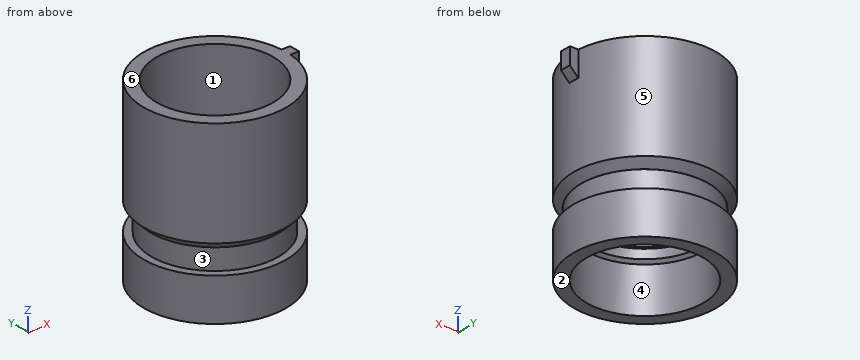
```python
from build123d import *

# Parameters (mm, degrees)
F0_R         = 17.1
F0_R_2       = 14
F1_DEPTH     = 10.2
F2_R         = 15.275
F2_R_2       = 14
F2_R_3       = 13.275
F3_DEPTH     = 5
F4_R         = 17.1
F4_R_2       = 15.275
F4_R_3       = 14
F5_DEPTH     = 27.1
F6_S5_R      = 14
F6_T6_DEPTH  = 22
F6_S11_R     = 14
F6_T12_DEPTH = 22
F7_SIZE      = 1.8
F9_DEPTH     = 6
F10_SIZE     = 1.99999


# Not quite as in the source:
# - a fillet or chamfer that OpenCascade refuses, or shapes differently, is made with other operations: its cross-section is extruded or revolved along the edge and cut away or added
# - a fillet or chamfer is up to 0.001 mm smaller than in the source, because OpenCascade refuses the exact size


with BuildPart() as f1:
    # F0 (on Top) → F1 (new body)
    with BuildSketch(Plane.XY):
        Circle(F0_R)
        Circle(F0_R_2, mode=Mode.SUBTRACT)
    extrude(amount=F1_DEPTH)

    # F2 (on face) → F3 (join)
    with BuildSketch(Plane.XY.offset(10.2)):
        Circle(F2_R)
        Circle(F2_R_2, mode=Mode.SUBTRACT)
        Circle(F2_R_2)
        Circle(F2_R_3, mode=Mode.SUBTRACT)
    extrude(amount=F3_DEPTH)

    # F4 (on face) → F5 (join)
    with BuildSketch(Plane.XY.offset(15.2)):
        Circle(F4_R)
        Circle(F4_R_2, mode=Mode.SUBTRACT)
        Circle(F4_R_2)
        Circle(F4_R_3, mode=Mode.SUBTRACT)
    extrude(amount=F5_DEPTH)

    # F6: chamfer of 1.4 on 2 edges, made by hand


with BuildPart() as f6_tool2:
    # F6_s3 → F6_t4 (revolve)
    with BuildSketch(Plane.XZ):
        Polygon((14.675, 10.2), (13.275, 11.6), (13.275, 10.2), align=None)
    revolve(axis=Axis((0, 0, 10.2), (0, 0, 1)))

    # F6_s5 → F6_t6 (intersect, symmetric)
    with BuildSketch(Plane.XY.offset(10.9)):
        Circle(F6_S5_R)
    extrude(amount=F6_T6_DEPTH, both=True, mode=Mode.INTERSECT)


with BuildPart() as f1_1:
    add(f1.part)

    # F6_t1: cut F6_tool2
    add(f6_tool2.part, mode=Mode.SUBTRACT)


with BuildPart() as f6_tool8:
    # F6_s9 → F6_t10 (revolve)
    with BuildSketch(Plane.XZ):
        Polygon((13.275, 13.8), (14.675, 15.2), (13.275, 15.2), align=None)
    revolve(axis=Axis((0, 0, 15.2), (0, 0, 1)))

    # F6_s11 → F6_t12 (intersect, symmetric)
    with BuildSketch(Plane.XY.offset(14.5)):
        Circle(F6_S11_R)
    extrude(amount=F6_T12_DEPTH, both=True, mode=Mode.INTERSECT)


with BuildPart() as f1_2:
    add(f1_1.part)

    # F6_t7: cut F6_tool8
    add(f6_tool8.part, mode=Mode.SUBTRACT)

    # F7
    f7_edges = [f1_2.edges().sort_by_distance(p)[0] for p in [
        (-17.1, 0, 15.2),
    ]]
    chamfer(f7_edges, length=F7_SIZE)

    # F8 (on face) → F9 (join)
    with BuildSketch(Plane.XY.offset(42.3)):
        with BuildLine():
            ThreePointArc((17.0505131888, 1.3), (17.0876238185, 0.6504707804), (17.1, 0))
            Line((17.1, 0), (19.1, 0))
            Line((19.1, 0), (19.1, 1.3))
            Line((19.1, 1.3), (17.0505131888, 1.3))
        make_face()
        with BuildLine():
            Line((19.1, 0), (17.1, 0))
            ThreePointArc((17.1, 0), (17.0876238185, -0.6504707804), (17.0505131888, -1.3))
            Line((17.0505131888, -1.3), (19.1, -1.3))
            Line((19.1, -1.3), (19.1, 0))
        make_face()
        with BuildLine():
            Line((17.1, 0), (17.0505131888, 0))
            Line((17.0505131888, 0), (17.0505131888, -1.3))
            ThreePointArc((17.0505131888, -1.3), (17.0876238185, -0.6504707804), (17.1, 0))
        make_face()
        with BuildLine():
            Line((17.0505131888, 1.3), (17.0505131888, 0))
            Line((17.0505131888, 0), (17.1, 0))
            ThreePointArc((17.1, 0), (17.0876238185, 0.6504707804), (17.0505131888, 1.3))
        make_face()
    extrude(amount=-F9_DEPTH)

    # F10 (size 2 in the source; OpenCascade refuses exactly that, so slightly less here)
    f10_edges = [f1_2.edges().sort_by_distance(p)[0] for p in [
        (19.1, 0, 36.3),
    ]]
    chamfer(f10_edges, length=F10_SIZE)


solid = f1_2.part
```
The model under review builds one solid part; all positions refer to its coordinate system, in mm. Face numbers are marked on the shaded views. A direction names the side the tool comes from. Round coordinates to 2 decimals unless told otherwise and drop trailing zeros. Loops run counter-clockwise (first coordinate to the right, second up) from the corner with the lowest first, then second, coordinate; pieces in that order, holes last. Notation, with made-up numbers: M 46,-14.75 L 60,-14.75 A26 ccw 60,22.25 Z; hole C -15.75,13 d1. An arc over 180 degrees is marked long. Put each result on its own line as item: value.
Q1. Machinability: for the marked faces 1, 2 and 3, which of the approach directions +Z, -Z, +X, -X, +Y, -Y give a long, thin tool a straight path to every point of the face, cutting with its end or side? Answer none if there is none.
Result set:
face 1: +Z
face 2: -Z, +X, -X, +Y, -Y
face 3: none
Q2. Consider section A-A, the plane x = 0. Give the boundary of the cut face in (y, z) (3 decimals), then the cut area to 3 significant figures.
Result set:
outline: M -17.1,0 L -14,0 L -14,10.875 L -13.275,11.6 L -13.275,13.8 L -14,14.525 L -14,42.3 L -17.1,42.3 L -17.1,17 L -15.3,15.2 L -15.275,15.2 L -15.275,10.2 L -17.1,10.2 Z; M 13.275,11.6 L 14,10.875 L 14,0 L 17.1,0 L 17.1,10.2 L 15.275,10.2 L 15.275,15.2 L 15.3,15.2 L 17.1,17 L 17.1,42.3 L 14,42.3 L 14,14.525 L 13.275,13.8 Z
area: 245 mm²
Q3. Mouldability with a two-part tool opening along Y and no side actions: class the marked faces 4, 5 and 6 as released by +Y, released by -Y, zero draft, split by the parting line, or undercut.
Result set:
face 4: undercut
face 5: split by the parting line
face 6: zero draft
Q4. To check wall thickness, follow L1, parallel to Y at x = 0, z = 35.75; L2, parallel to Y at x = 0, z = 12 (3 decimals); L3, parallel to X at y = -5.5, z = 38. State the ranges of each line that lie inside material, in increasing order.
Result set:
L1: y = -17.1 to -14, 14 to 17.1
L2: y = -15.275 to -13.275, 13.275 to 15.275
L3: x = -16.19 to -12.87, 12.87 to 16.19
Q5. For pin 1 (0.6 mm diameter, centred on x = 18, z = 39.5, fed in from +Y); pin 2 (8 mm diameter, centred on x = 6, y = 7.5, fed in from -Z); pin 3 (1.6 mm diameter, centred on x = 18.5, z = 40, fed in from -Y); pin 4 (9 mm diameter, centred on x = 5.5, y = -0.5, fed in from -Z), all flat-tipped, find the tip position at first contact; note any pin that passes through.
Result set:
pin 1: stops at y = 1.3
pin 2: stops at z = 11.27
pin 3: stops at y = -1.3
pin 4: passes through
Q6. Consider section B-B, the plane z = 3. Give the boundary of the cut face in (x, y).
Result set:
outline: C 0,0 d34.2; hole C 0,0 d28
